For this review, take the finished solid that the model builds, in its own axes (mm). A direction names the side the tool comes from. Coordinates: 2 decimals unless noted, no trailing zeros. Order: outer loops, then holes, each group sorted by start corner. A loop starts at its lowest first (then second) coordinate and runs counter-clockwise, first axis right, second up. Notation, with made-up numbers: (-38, -6.5) -> (-23, -6.5) arc R32 cw to (-23, 20.5) -> close; hole circle Ø1 at (17.5, 60.5). An arc over 180 degrees is marked (long way). Return JSON: item names as keys, results as strings. Group by question number.
Item 1: Take a section at B-B (x = 83.5). Write out the cut boundary in (y, z).
Item 2: For line 1 along Y through (x, z) = (1, 6); line 2 along X through (y, z) = (108, 6.75), list the stretches that pass through material, from the lowest coordinate up.
Item 3: Insertion check: pin 1 (2.5 mm diameter, centred on y = 115.5, z = 3.5, fed in from -X); pin 2 (4 mm diameter, centred on x = -1, z = 6, fed in from +Y); pin 3 (2.5 mm diameter, centred on y = -94, z = 2.5, fed in from +X). Each pin has a flat end and moves straight along its axis. Give the tip position at first contact, or say it passes through.
Item 4: Take a section at C-C (y = -94). Write out the cut boundary in (x, z).
Item 5: Take a section at A-A (z = 4.5). Write out the cut boundary in (x, y).
Item 6: Machinability: for faces 1 (the flat face through (-101, -87.5, 4)), 2 (the flat face through (-21, 116, 4)), 3 (the flat face through (-63, 117, 4)), which of the approach directions +Z, -Z, +X, -X, +Y, -Y give a long, thin tool a straight path to every point of the face, cutting with its end or side? Answer none if there is none.
Item 7: Draft analysis for pull direction X (two halves, no side actions). For faces 4 (the flat face through (21, 116, 4)), 5 (the flat face through (0, 112.5, 4)), 6 (the flat face through (-1, 6, 0)), 7 (the flat face through (97, -100, 4)), state which applies: +X half, -X half, draft (parallel to the pull), parting line (faces both ways), or undercut.
Autodesk Inventor part; units mm, degrees
ref_plane "YZ Plane" through (0, 0, 0) normal (1, 0, 0) x (0, 1, 0)
ref_plane "XZ Plane" through (0, 0, 0) normal (0, 1, 0) x (-1, 0, 0)
ref_plane "XY Plane" through (0, 0, 0) normal (0, 0, 1) x (1, 0, 0)
sketch "Sketch2" plane through (0, 0, 0) normal (0, 0, 1) x (1, 0, 0)
  line L0 (-105, -112.5) -> (105, -112.5)
  line L1 (105, -112.5) -> (105, 112.5)
  line L2 (105, 112.5) -> (-105, 112.5)
  line L3 (-105, 112.5) -> (-105, -112.5)
  line L4 (-105, -112.5) -> (105, 112.5) construction
  line L5 (105, -112.5) -> (-105, 112.5) construction
  point P0 (0, 0)
  dimension "d11" = 225
  dimension "d12" = 210
extrude "Extrusion2" add sketch "Sketch2" along normal blind 8
sketch "Sketch3" plane through (0, 0, 8) normal (0, 0, 1) x (1, 0, 0)
  line L0 (105, 112.5) -> (-105, 112.5)
  line L1 (-63, 112.5) -> (-21, 112.5)
  line L2 (-21, 112.5) -> (-21, 120.5)
  line L3 (-21, 120.5) -> (-63, 120.5)
  line L4 (-63, 120.5) -> (-63, 112.5)
  line L5 (63, 112.5) -> (21, 112.5)
  line L6 (21, 112.5) -> (21, 120.5)
  line L7 (21, 120.5) -> (63, 120.5)
  line L8 (63, 120.5) -> (63, 112.5)
  line L9 (-21, 120.5) -> (21, 120.5) construction
  line L10 (63, 120.5) -> (105, 120.5) construction
  line L11 (-63, 120.5) -> (-105, 120.5) construction
  point P0 (0, 0)
  dimension "d15" = 8
extrude "Extrusion3" add sketch "Sketch3" against normal blind 8
sketch "Sketch4" plane through (0, 0, 8) normal (0, 0, 1) x (1, 0, 0)
  line L0 (-105, 112.5) -> (-105, -112.5)
  line L1 (-105, -112.5) -> (-97, -112.5)
  line L2 (-97, -112.5) -> (-97, -87.5)
  line L3 (-97, -87.5) -> (-105, -87.5)
  line L4 (-105, -87.5) -> (-105, -112.5)
  line L5 (-105, 112.5) -> (-97, 112.5)
  line L6 (-97, 112.5) -> (-97, 87.5)
  line L7 (-97, 87.5) -> (-105, 87.5)
  line L8 (-105, 87.5) -> (-105, 112.5)
  line L9 (-97, -87.5) -> (-97, 87.5) construction
  point P0 (0, 0)
  dimension "d21" = 8
  dimension "d22" = 25
extrude "Extrusion4" cut sketch "Sketch4" against normal blind 8
mirror "Mirror2" about plane through (0, 0, 0) normal (1, 0, 0) of "Extrusion4"
properties part number "M06 - Wall Side 1" material "Polycarbonate, Clear"
Findings below:
{
 "1": {"outline": "(-112.5, 0) -> (112.5, 0) -> (112.5, 8) -> (-112.5, 8) -> close"},
 "2": {"line 1": "y = -112.5 to 112.5", "line 2": "x = -97 to 97"},
 "3": {"pin 1": "stops at x = -63", "pin 2": "stops at y = 112.5", "pin 3": "stops at x = 97"},
 "4": {"outline": "(-97, 0) -> (97, 0) -> (97, 8) -> (-97, 8) -> close"},
 "5": {"outline": "(-105, -87.5) -> (-97, -87.5) -> (-97, -112.5) -> (97, -112.5) -> (97, -87.5) -> (105, -87.5) -> (105, 87.5) -> (97, 87.5) -> (97, 112.5) -> (63, 112.5) -> (63, 120.5) -> (21, 120.5) -> (21, 112.5) -> (-21, 112.5) -> (-21, 120.5) -> (-63, 120.5) -> (-63, 112.5) -> (-97, 112.5) -> (-97, 87.5) -> (-105, 87.5) -> close"},
 "6": {"face 1": "+Z, -Z, -X, -Y", "face 2": "+Z, -Z, +Y", "face 3": "+Z, -Z, -X, +Y"},
 "7": {"face 4": "undercut", "face 5": "undercut", "face 6": "draft", "face 7": "+X half"}
}
